Model file for the job. Use its own axes, mm. A direction names the side the tool comes from. Coordinates: 2 decimals unless noted, no trailing zeros. Order: outer loops, then holes, each group sorted by start corner. A loop starts at its lowest first (then second) coordinate and runs counter-clockwise, first axis right, second up.
from build123d import *
from OCP.BRepFilletAPI import BRepFilletAPI_MakeChamfer

# Parameters (mm, degrees)
EXTRUDE1_DEPTH                                   = 342.9
CHAMFER1_SIZE                                    = 19.05
CHAMFER1_SIZE2                                   = 5.104432116
CHAMFER3_SIZE                                    = 19.05
CHAMFER3_SIZE2                                   = 5.104432116
CBORE_FOR_1_4_SOCKET_HEAD_CAP_SCREW1_D           = 6.7564
CBORE_FOR_1_4_SOCKET_HEAD_CAP_SCREW1_CBORE_D     = 11.1125
CBORE_FOR_1_4_SOCKET_HEAD_CAP_SCREW1_CBORE_DEPTH = 16.51
C_0_242_DIAMETER_HOLE1_D                         = 6.1468


with BuildPart() as part:
    # Sketch1 → Extrude1 (new, symmetric)
    with BuildSketch(Plane.XY):
        Polygon((0, 0), (0, 22.225), (-15.875, 22.225), (-15.875, 9.525), (-41.275, 9.525), (-41.275, 0), (-28.448, 0), align=None)
    extrude(amount=EXTRUDE1_DEPTH, both=True)

    # Chamfer1: one chamfer whose edges measure the first distance from different faces: ONE call of the kernel's chamfer builder (chamfer() names one face for all edges)
    chamfer1_edges_1 = [part.edges().sort_by_distance(p)[0] for p in [
        (-28.575, 9.525, 342.9),
    ]]
    chamfer1_side_1 = [part.faces().sort_by_distance(p)[0] for p in [
        (-28.575, 9.525, 0),
    ]]
    chamfer1_edges_2 = [part.edges().sort_by_distance(p)[0] for p in [
        (-15.875, 15.875, 342.9),
    ]]
    chamfer1_side_2 = [part.faces().sort_by_distance(p)[0] for p in [
        (-15.875, 15.875, 0),
    ]]
    chamfer1 = BRepFilletAPI_MakeChamfer(part.part.solid().wrapped)
    for e in chamfer1_edges_1:
        chamfer1.Add(CHAMFER1_SIZE, CHAMFER1_SIZE2, e.wrapped, chamfer1_side_1[0].wrapped)  # the first distance lies on this face
    for e in chamfer1_edges_2:
        chamfer1.Add(CHAMFER1_SIZE, CHAMFER1_SIZE2, e.wrapped, chamfer1_side_2[0].wrapped)  # the first distance lies on this face
    add(Compound.cast(chamfer1.Shape()), mode=Mode.REPLACE)

    # Chamfer3: one chamfer whose edges measure the first distance from different faces: ONE call of the kernel's chamfer builder (chamfer() names one face for all edges)
    chamfer3_edges_1 = [part.edges().sort_by_distance(p)[0] for p in [
        (-15.875, 15.875, -342.9),
    ]]
    chamfer3_side_1 = [part.faces().sort_by_distance(p)[0] for p in [
        (-15.875, 15.875, -9.525),
    ]]
    chamfer3_edges_2 = [part.edges().sort_by_distance(p)[0] for p in [
        (-28.575, 9.525, -342.9),
    ]]
    chamfer3_side_2 = [part.faces().sort_by_distance(p)[0] for p in [
        (-28.575, 9.525, -9.525),
    ]]
    chamfer3 = BRepFilletAPI_MakeChamfer(part.part.solid().wrapped)
    for e in chamfer3_edges_1:
        chamfer3.Add(CHAMFER3_SIZE, CHAMFER3_SIZE2, e.wrapped, chamfer3_side_1[0].wrapped)  # the first distance lies on this face
    for e in chamfer3_edges_2:
        chamfer3.Add(CHAMFER3_SIZE, CHAMFER3_SIZE2, e.wrapped, chamfer3_side_2[0].wrapped)  # the first distance lies on this face
    add(Compound.cast(chamfer3.Shape()), mode=Mode.REPLACE)

    # CBORE for 1/4 Socket Head Cap Screw1 (through all)
    with Locations(Plane(origin=(0, 22.225, 0), x_dir=(-1, 0, 0), z_dir=(0, 1, 0))):
        with Locations((7.112, 304.8), (7.112, -304.8)):
            CounterBoreHole(CBORE_FOR_1_4_SOCKET_HEAD_CAP_SCREW1_D / 2, CBORE_FOR_1_4_SOCKET_HEAD_CAP_SCREW1_CBORE_D / 2, CBORE_FOR_1_4_SOCKET_HEAD_CAP_SCREW1_CBORE_DEPTH)

    # C (0.242) Diameter Hole1 (through all)
    with Locations(Plane(origin=(2.077199123, 9.525, 2.74697932), x_dir=(1, 0, 0), z_dir=(0, 1, 0))):
        with Locations((-22.651199123, -261.52541668), (-22.651199123, 267.01937532)):
            Hole(C_0_242_DIAMETER_HOLE1_D / 2)


solid = part.part
Q1. Cut at A-A, the plane y = 15.5. Count the separate pieces of the cut face and the enclosed holes in it, plus the area to 3 significant figures.
Established:
separate pieces: 1
enclosed holes: 2
area: 10,600 mm2
Q2. Probe line 1 (Z direction, x = -6.5, y = 8); line 2 (Z direction, x = -7, y = 21); line 3 (X direction, y = 12, z = 304.8) (3 decimals). List the from-to ranges inside material, lowest first.
Established:
line 1: z = -342.9 to -310.32, -299.28 to 299.28, 310.32 to 342.9
line 2: z = -342.9 to -310.36, -299.24 to 299.24, 310.36 to 342.9
line 3: x = -15.875 to -12.668, -1.556 to 0
Q3. Mould opens along Z. For faces 6 (the face through (-12, 4, 342.9)), 7 (the face through (-15.875, 16, 5)), 8 (the face through (-12, 4, -342.9)), 9 (the face through (-9.676, 14.086, -309.729)) say: pulls with the +Z half, pulls with the -Z half, needs draft (parallel to the pull), parting line crosses it, or undercut.
Established:
face 6: pulls with the +Z half
face 7: needs draft
face 8: pulls with the -Z half
face 9: undercut
Q4. Cut at B-B, the plane z = -114. List the corners of the cut face in (x, y) (3 decimals), plus the area to 3 significant figures.
Established:
outline: (-41.275, 0) - (0, 0) - (0, 22.225) - (-15.875, 22.225) - (-15.875, 9.525) - (-41.275, 9.525) - close
area: 595 mm2
Q5. Which spindle directions (+Z, -Z, +X, -X, +Y, -Y) get a long thin tool onto all of the face, cutting with end or side? Do faces 1 (the face through (-28, 9.525, 5)), 2 (the face through (-21, 0, 5)), 3 (the face through (-25.809, 6.937, -333.508)), 4 (the face through (-25.809, 6.937, 333.508)), 5 (the face through (-10, 5.715, -307)). Say none if no direction does.
Established:
face 1: +Z, -Z, -X, +Y
face 2: +Z, -Z, +X, -X, -Y
face 3: -Z, -X, +Y
face 4: +Z, -X, +Y
face 5: +Y
Q6. Drop flat-ended pins along their axis: P1, Ø7, axis at x = -20.57, z = 264.27, coming from the +Y side (3 decimals); P2, Ø1.5, axis at y = 14.5, z = -80.5, coming from the -X side (3 decimals); P3, Ø6, axis at x = -7.112, z = 304.8, coming from the +Y side; P4, Ø5.5, axis at x = -8.5, z = -302.5, coming from the +Y side (3 decimals). Give the stop position or say it passes through.
Established:
P1: stops at y = 9.525
P2: stops at x = -15.875
P3: passes through
P4: stops at y = 5.715
